from build123d import *

# Parameters (mm, degrees)
F1_DEPTH = 25.4
F2_DEPTH = 31.75


with BuildPart() as f1:
    # F0 (on Top) → F1 (new body)
    with BuildSketch(Plane.XY):
        Polygon((0, 25.4), (0, 0), (12.7, 0), (12.7, 25.4), (19.05, 25.4), (19.05, 38.1), (-6.35, 38.1), (-6.35, 25.4), align=None)
    extrude(amount=F1_DEPTH)

    # F1_face (on face) → F2 (join)
    with BuildSketch(Plane(origin=(6.35, 22.225, 25.4), x_dir=(1, 0, 0), z_dir=(0, 0, 1))):
        Polygon((-12.7, 3.175), (-6.35, 3.175), (-6.35, -22.225), (6.35, -22.225), (6.35, 3.175), (12.7, 3.175), (12.7, 15.875), (-12.7, 15.875), align=None)
    extrude(amount=F2_DEPTH)


solid = f1.part
Could you check a few things on this model? Use its own coordinates, in mm. A direction names the side the tool comes from. Give positions to 0.01 mm unless a question says otherwise; leave off trailing zeros. Order: outer loops, then holes, each group sorted by start corner. A loop starts at its lowest first (then second) coordinate and runs counter-clockwise, first axis right, second up. Notation, with made-up numbers: (-10.5, 84) -> (29.5, 84) arc R20 cw to (29.5, 104) -> close; hole circle Ø9 at (12.5, 79). An arc over 180 degrees is marked (long way). Return JSON: item names as keys, results as strings.
1. Imagine slicing it at A-A on z = 14.5. List the corners of the cut face in (x, y) for me.
Answer list:
{"outline": "(-6.35, 25.4) -> (0, 25.4) -> (0, 0) -> (12.7, 0) -> (12.7, 25.4) -> (19.05, 25.4) -> (19.05, 38.1) -> (-6.35, 38.1) -> close"}
2. I need wall thicknesses on line 1 (Y direction, x = 17.5, z = 14.5); line 2 (X direction, y = 2, z = 9.5). Which ranges of each line are inside material? Lowest first, please. Write a range as from..to.
Answer list:
{"line 1": "y = 25.4..38.1", "line 2": "x = 0..12.7"}
3. Thinking about a two-plate mould opening in Y: for faces 4 (the flat face through (0, 13, 28)), 5 (the flat face through (7, 38.1, 28)), 6 (the flat face through (6, 0, 28)), which applies, pulls with the +Y half, pulls with the -Y half, needs draft (parallel to the pull), parting line crosses it, or undercut?
Answer list:
{"face 4": "needs draft", "face 5": "pulls with the +Y half", "face 6": "pulls with the -Y half"}
4. On a 3-axis mill with a long thin cutter (end or side, diameter ignored), from which of +Z, -Z, +X, -X, +Y, -Y can I reach the whole of each face in a straight line? I mean faces 1 (the flat face through (12.7, 13, 28)), 2 (the flat face through (-3, 25.4, 28)), 3 (the flat face through (6, 24, 57.15)). Say none if no direction works.
Answer list:
{"face 1": "+Z, -Z, +X, -Y", "face 2": "+Z, -Z, -X, -Y", "face 3": "+Z, +X, -X, +Y, -Y"}
5. Imagine slicing it at C-C on y = 13.5. List the corners of the cut face in (x, z) for me.
Answer list:
{"outline": "(0, 0) -> (12.7, 0) -> (12.7, 57.15) -> (0, 57.15) -> close"}
6. For pin 1 Ø6 at (y, z) = (12.5, 22) entering from -X; pin 2 Ø3 at (x, z) = (15, 15.5) entering from -Y; pin 3 Ø12.5 at (y, z) = (14, 34.5) entering from +X, each with a flat end and sliding along its axis, tell me the tip position at first contact or that it passes through.
Answer list:
{"pin 1": "stops at x = 0", "pin 2": "stops at y = 25.4", "pin 3": "stops at x = 12.7"}
7. Imagine slicing it at B-B on x = -3. List the corners of the cut face in (y, z) for me, then the cut area to 3 significant figures.
Answer list:
{"outline": "(25.4, 0) -> (38.1, 0) -> (38.1, 57.15) -> (25.4, 57.15) -> close", "area": "726 mm2"}
